Can you work these out from the model? Positions are in its coordinate system, mm. Face numbers are marked on the shaded views. A direction names the side the tool comes from. Coordinates: 2 decimals unless noted, no trailing zeros. Order: outer loops, then holes, each group sorted by start corner. A loop starts at its lowest first (then second) coordinate and runs counter-clockwise, first axis right, second up.
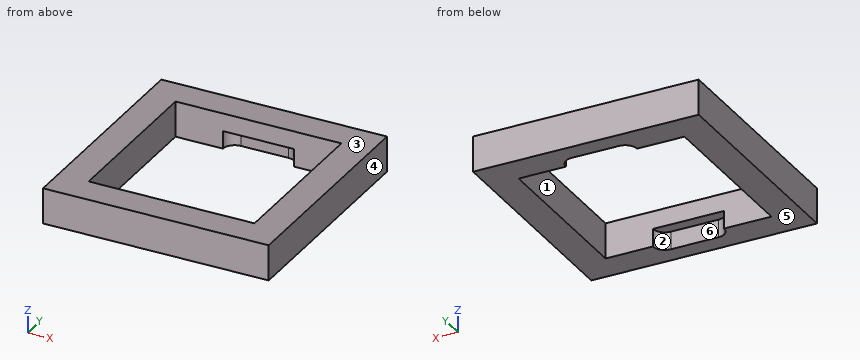
Autodesk Fusion 360 part; units mm, degrees
sketch "スケッチ1" plane through (0, 0, 0) normal (0, 0, 1) x (1, 0, 0)
  line L0 (7, -7) -> (-7, -7)
  line L1 (-7, -7) -> (-7, 7)
  line L2 (-7, 7) -> (7, 7)
  line L3 (7, 7) -> (7, -7)
  line L4 (9.525, -9.525) -> (-9.525, -9.525)
  line L5 (-9.525, -9.525) -> (-9.525, 9.525)
  line L6 (-9.525, 9.525) -> (9.525, 9.525)
  line L7 (9.525, 9.525) -> (9.525, -9.525)
  line L8 (3, 7) -> (3, 7)
  line L9 (-3, 7) -> (-3, 7)
  line L10 (-2, 8) -> (2, 8)
  line L11 (3, -7) -> (3, -7)
  line L12 (2, -8) -> (-2, -8)
  line L13 (-3, -7) -> (-3, -7)
  arc A0 (2, -8) -> (3, -7) centre (2, -7) ccw
  arc A1 (-3, -7) -> (-2, -8) centre (-2, -7) ccw
  arc A2 (3, 7) -> (2, 8) centre (2, 7) ccw
  arc A3 (-2, 8) -> (-3, 7) centre (-2, 7) ccw
  dimension "d8" = 1
extrude "押し出し1" add sketch "スケッチ1" along normal blind 3
extrude "押し出し2" add sketch "スケッチ1" along normal blind 1.5 from surface at 1.5 contours L0 L12 A0 A1 | L2 L10 A2 A3
1. Imagine slicing it at C-C on z = 2.1. Please give me the cut outline in (x, y) (3 decimals), then the cut area to 3 significant figures.
Completed:
outline: (-9.525, -9.525) - (9.525, -9.525) - (9.525, 9.525) - (-9.525, 9.525) - close; hole (-7, -7) - (7, -7) - (7, 7) - (-7, 7) - close
area: 167 mm2
2. I'm going to push flat-ended pins straight in: pin 1 (3 mm diameter, centred on x = -6.5, y = 6, fed in from +Z); pin 2 (0.5 mm diameter, centred on x = 0.5, y = -7.5, fed in from -Z). Where does each tip first touch, or does it pass through?
Completed:
pin 1: stops at z = 3
pin 2: stops at z = 1.5
3. Please list where this line runs through material, in increasing order: probe 1 along Y at (x, z) = (6.75, 2.5) (3 decimals).
Completed:
probe 1: y = -9.525 to -7, 7 to 9.525
4. On a 3-axis mill with a long thin cutter (end or side, diameter ignored), from which of +Z, -Z, +X, -X, +Y, -Y can I reach the whole of each face in a straight line? I mean the marked faces 1, 2 and 3. Say none if no direction works.
Completed:
face 1: +Z, -Z
face 2: -Z
face 3: +Z, +X, -X, +Y, -Y
5. Imagine slicing it at A-A on x = -1.5. Please give me the cut outline in (y, z) (3 decimals), then the cut area to 4 significant figures.
Completed:
outline: (-9.525, 0) - (-8, 0) - (-8, 1.5) - (-7, 1.5) - (-7, 3) - (-9.525, 3) - close; (7, 1.5) - (8, 1.5) - (8, 0) - (9.525, 0) - (9.525, 3) - (7, 3) - close
area: 12.15 mm2
6. Imagine slicing it at B-B on y = 2. Please give me the cut outline in (x, z) (3 decimals), then the cut area to 4 significant figures.
Completed:
outline: (-9.525, 0) - (-7, 0) - (-7, 3) - (-9.525, 3) - close; (7, 0) - (9.525, 0) - (9.525, 3) - (7, 3) - close
area: 15.15 mm2
7. Thinking about a two-plate mould opening in X: for the marked faces 4, 5 and 6, which applies, pulls with the +X half, pulls with the -X half, needs draft (parallel to the pull), parting line crosses it, or undercut?
Completed:
face 4: pulls with the +X half
face 5: needs draft
face 6: undercut
8. Imagine slicing it at D-D on z = 0.8. Please give me the cut outline in (x, y) (3 decimals), then the cut area to 3 significant figures.
Completed:
outline: (-9.525, -9.525) - (9.525, -9.525) - (9.525, 9.525) - (-9.525, 9.525) - close; hole (-7, -7) - (-3, -7) arc R1 ccw to (-2, -8) - (2, -8) arc R1 ccw to (3, -7) - (7, -7) - (7, 7) - (3, 7) arc R1 ccw to (2, 8) - (-2, 8) arc R1 ccw to (-3, 7) - (-7, 7) - close
area: 156 mm2
